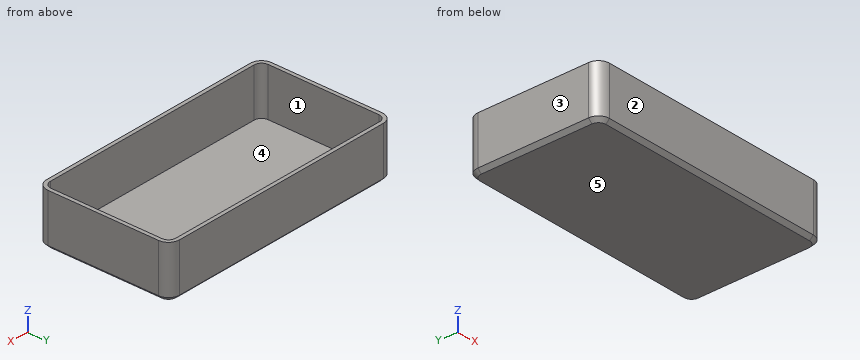
```python
from build123d import *

# Parameters (mm, degrees)
PAD_DEPTH    = 14
THICKNESS_T  = -1
CHAMFER_SIZE = 1


with BuildPart() as part:
    # Sketch → Pad (new body)
    with BuildSketch(Plane.XY):
        with BuildLine():
            Line((0, 3), (0, 33))
            ThreePointArc((3, 36), (0.87868, 35.12132), (0, 33))
            Line((3, 36), (65, 36))
            ThreePointArc((68, 33), (67.12132, 35.12132), (65, 36))
            Line((68, 33), (68, 3))
            ThreePointArc((65, 0), (67.12132, 0.87868), (68, 3))
            Line((3, 0), (65, 0))
            ThreePointArc((0, 3), (0.87868, 0.87868), (3, 0))
        make_face()
    extrude(amount=PAD_DEPTH)

    # Thickness
    thickness_openings = [part.faces().sort_by_distance(p)[0] for p in [
        (34, 18, 14),
    ]]
    offset(amount=THICKNESS_T, openings=thickness_openings)

    # Chamfer
    chamfer_edges = [part.edges().sort_by_distance(p)[0] for p in [
        (34, 0, 0),
    ]]
    chamfer(chamfer_edges, length=CHAMFER_SIZE)


solid = part.part
```
Work out the finished part from the listing and answer in its coordinate system (mm). Face numbers are marked on the shaded views. A direction names the side the tool comes from. Give positions to 0.01 mm unless a question says otherwise; leave off trailing zeros. Loops run counter-clockwise (first coordinate to the right, second up) from the corner with the lowest first, then second, coordinate; pieces in that order, holes last. Notation, with made-up numbers: M -22.75,40 L 30.25,40 A16 cw 30.25,59 Z; hole C 83.25,21 d10. An arc over 180 degrees is marked long. One line per item, written item: value. Start each with the question number.
1. Find section A-A (x = 63). Give the vertices of the cut face in (y, z).
2. Find section C-C (y = 14). Give the vertices of the cut face in (x, z).
3. This flat-tipped pin is pushed along its axis until it touches: P1, Ø1.5, axis at x = 46.5, y = 18.5, coming from the +Z side. Where does it stop, or does it pass through?
4. Which of the six approach directions +Z, -Z, +X, -X, +Y, -Y give full straight-line access (tool end or side, diameter ignored) to the marked faces 4 and 5?
5. Determine the mould class of the marked faces 1, 2 and 3 for opening direction X: released by +X, released by -X, zero draft, split by the parting line, or undercut.
6. Find section B-B (z = 13). Give the vertices of the cut face in (x, y).
7. Find the intervals of material crossed by probe 1 along Y at (x, z) = (45, 12.5); probe 2 along X at (y, z) = (30, 5.5); probe 3 along Z at (x, y) = (46, 24.5), in increasing order.
Reported:
1. outline: M 0,1 L 1,0 L 35,0 L 36,1 L 36,14 L 35,14 L 35,1 L 1,1 L 1,14 L 0,14 Z
2. outline: M 0,1 L 1,0 L 67,0 L 68,1 L 68,14 L 67,14 L 67,1 L 1,1 L 1,14 L 0,14 Z
3. P1: stops at z = 1
4. face 4: +Z
4. face 5: -Z, +X, -X, +Y, -Y
5. face 1: undercut
5. face 2: zero draft
5. face 3: released by -X
6. outline: M 0,3 A3 ccw 3,0 L 65,0 A3 ccw 68,3 L 68,33 A3 ccw 65,36 L 3,36 A3 ccw 0,33 Z; hole M 1,3 A2 ccw 3,1 L 65,1 A2 ccw 67,3 L 67,33 A2 ccw 65,35 L 3,35 A2 ccw 1,33 Z
7. probe 1: y = 0 to 1, 35 to 36
7. probe 2: x = 0 to 1, 67 to 68
7. probe 3: z = 0 to 1
